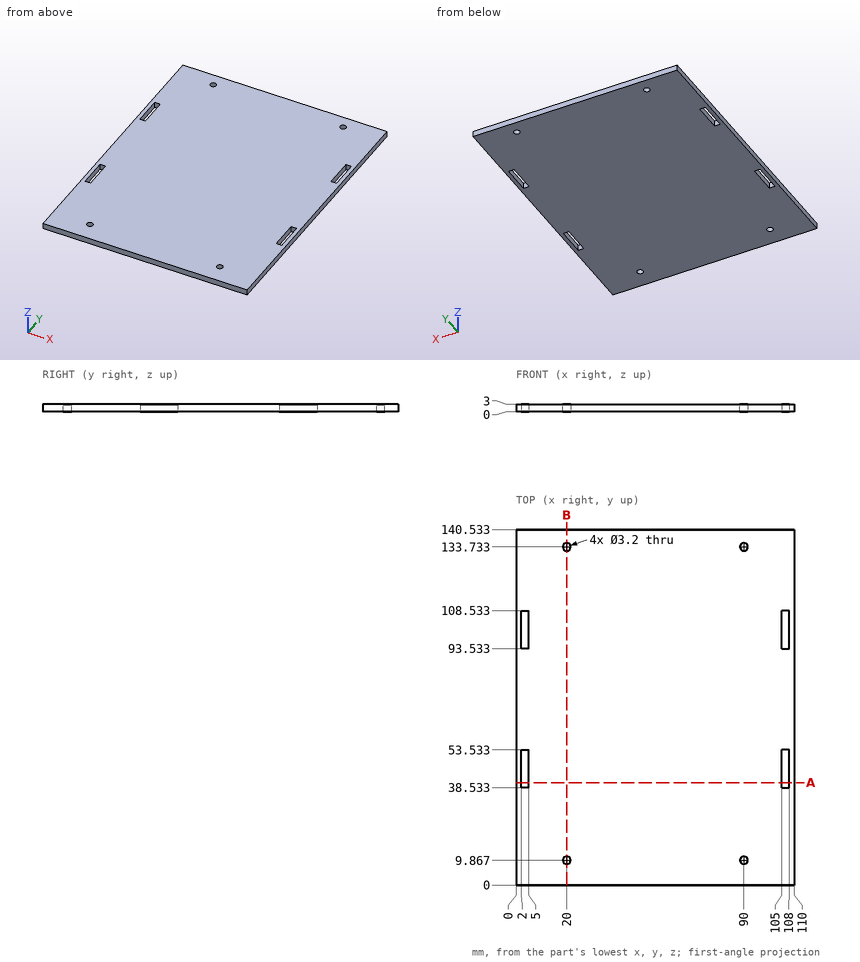
Geometry: see drawing. Coordinates: mm, zero at the bounding-box minimum. Give positions to 0.01 mm unless a question says otherwise; leave off trailing zeros. Order: outer loops, then holes, each group sorted by start corner. A loop starts at its lowest first (then second) coordinate and runs counter-clockwise, first axis right, second up. Notation, with made-up numbers: (69.5, -24.5) -> (83.5, -24.5) arc R30 ccw to (83.5, -0.5) -> close; hole circle Ø10 at (-35, 30). An arc over 180 degrees is marked (long way). Write item = value, one per line.
Q1. Cut plane B-B, the plane x = 20. Output: boundary loops of the cut face in (y, z).
Data:
outline = (0, 0) -> (8.27, 0) -> (8.27, 3) -> (0, 3) -> close; (11.47, 0) -> (132.13, 0) -> (132.13, 3) -> (11.47, 3) -> close; (135.33, 0) -> (140.53, 0) -> (140.53, 3) -> (135.33, 3) -> close
Q2. Pin query (flat end, axial travel): pin 1 (1.5 mm diameter, centred on x = 3, z = 1.5, fed in from -Y); pin 2 (3 mm diameter, centred on x = 90, y = 9.87, fed in from +Z). Return the tip coordinate at first contact, or that it passes through.
Data:
pin_1 = 0
pin_2 = through
Q3. Material intervals for line 1 (Y direction, x = 90, z = 1.4); line 2 (X direction, y = 47, z = 1.85); line 3 (X direction, y = 8.5, z = 2.1), sorted ascending. Write a range as from..to.
Data:
line_1 = 0..8.27, 11.47..132.13, 135.33..140.53
line_2 = 0..2, 5..105, 108..110
line_3 = 0..19.17, 20.83..89.17, 90.83..110
Q4. Cut plane A-A, the plane y = 40.5. Output: boundary loops of the cut face in (x, z).
Data:
outline = (0, 0) -> (2, 0) -> (2, 3) -> (0, 3) -> close; (5, 0) -> (105, 0) -> (105, 3) -> (5, 3) -> close; (108, 0) -> (110, 0) -> (110, 3) -> (108, 3) -> close
